Check sheet for the modelled part. Datum: model origin and axes. Units: mm. Give positions to 0.01 mm unless a question says otherwise; leave off trailing zeros. Write each loop counter-clockwise with the first axis right and the second up, starting at its lowest first coordinate (ties: lowest second). Pieces come first, ordered by that corner, then holes. Notation, with made-up numbers: M -27,87 L -18,87 A3 ccw -18,92 Z; hole C 73.5,-17 d3. An arc over 180 degrees is marked long. Write item = value, one per line. Start each with the question number.
1) Gauge pin test, flat end, axial feed: pin 1 (4 mm diameter, centred on x = 60.325, z = -53.975, fed in from +Y). Record the tip position at first contact, or that the pin passes through.
2) Scan lines: L1, parallel to Z at x = 60.5, y = -3 (3 decimals); L2, parallel to X at y = -1, z = -8. Record each from-to range of solid material in increasing order.
3) Draft check along Z on faces 1 (the face through (91, -4, -66.675)), 2 (the face through (62.35, -3.22, -52.42)), 3 (the face through (92.29, -3.78, -33.8)), 4 (the face through (91, -4, 0)). Enter one of: pulls with the +Z half, pulls with the -Z half, needs draft (parallel to the pull), parting line crosses it, or undercut.
4) Sectioned sample at B-B, the plane z = -12.7. Record the cut outline in (x, y) (3 decimals), then the cut area to 3 significant figures.
5) Sectioned sample at C-C, the plane z = -59. Record the cut outline in (x, y) (3 decimals), then the cut area to 3 significant figures.
6) Sectioned sample at A-A, the plane y = -2.5. Count the separate pieces of the cut face and the enclosed holes in it, then the cut area to 3 significant figures.
from build123d import *
from build123d.topology import SkipClean

# Parameters (mm, degrees)
SKETCH1_W              = 184.15
SKETCH1_H              = 66.675
BOSS_EXTRUDE1_DEPTH    = 10.541
SKETCH4_W              = 76.2
SKETCH4_H              = 6.35
BOSS_EXTRUDE2_DEPTH    = 66.675
SKETCH5_W              = 53.975
SKETCH5_H              = 66.675
CUT_EXTRUDE1_DEPTH     = 9.525
SKETCH17_W             = 53.975
SKETCH17_H             = 6.35
BOSS_EXTRUDE3_DEPTH    = 66.675
F_10_CLEARANCE_HOLE1_D = 5.1054
SKETCH12_R             = 31.019294643
CUT_EXTRUDE3_DEPTH     = 197.132329834
SKETCH18_W             = 53.975
SKETCH18_H             = 6.35
BOSS_EXTRUDE4_DEPTH    = 66.675
SKETCH20_W             = 53.975
SKETCH20_H             = 1.016
CUT_EXTRUDE8_DEPTH     = 197.132329834
SKETCH21_R             = 2.5527
CUT_EXTRUDE9_DEPTH     = 197.132329834
SKETCH22_W             = 184.15
SKETCH22_H             = 10.541
CUT_EXTRUDE10_DEPTH    = 197.132329834


with BuildPart() as part:
    # Sketch1 → Boss-Extrude1 (new body)
    with BuildSketch(Plane(origin=(0, 0, 0), x_dir=(1, 0, 0), z_dir=(0, 1, 0))):
        with Locations((92.075, 33.3375)):
            Rectangle(SKETCH1_W, SKETCH1_H)
    extrude(amount=BOSS_EXTRUDE1_DEPTH)

    # Sketch4 → Boss-Extrude2 (add)
    with BuildSketch(Plane.XY):
        with Locations((92.075, -3.175)):
            Rectangle(SKETCH4_W, SKETCH4_H)
    extrude(amount=-BOSS_EXTRUDE2_DEPTH)

    # Sketch5 → Cut-Extrude1 (cut)
    with BuildSketch(Plane(origin=(0, 10.541, 0), x_dir=(1, 0, 0), z_dir=(0, 1, 0))):
        with Locations((92.075, 33.3375)):
            Rectangle(SKETCH5_W, SKETCH5_H)
    extrude(amount=-CUT_EXTRUDE1_DEPTH, mode=Mode.SUBTRACT)

    # Sketch17 → Boss-Extrude3 (add)
    with BuildSketch(Plane.XY):
        with Locations((157.1625, -3.175)):
            Rectangle(SKETCH17_W, SKETCH17_H)
    extrude(amount=-BOSS_EXTRUDE3_DEPTH)

    # #10 Clearance Hole1 (through all)
    with Locations(Plane(origin=(0, 10.541, 0), x_dir=(1, 0, 0), z_dir=(0, 1, 0))):
        with Locations((9.525, 53.975), (9.525, 12.7), (60.325, 12.7), (60.325, 53.975), (123.825, 53.975), (123.849810746, 12.7), (174.625, 12.7), (174.625, 53.975)):
            Hole(F_10_CLEARANCE_HOLE1_D / 2)

    # Sketch12 → Cut-Extrude3 (cut, through all)
    with BuildSketch(Plane(origin=(0, 0, -66.675), x_dir=(-1, 0, 0), z_dir=(0, 0, -1))):
        with Locations((-92.075, 27.239371317)):
            Circle(SKETCH12_R)
    extrude(amount=-CUT_EXTRUDE3_DEPTH, mode=Mode.SUBTRACT)

    # Sketch18 → Boss-Extrude4 (add)
    with BuildSketch(Plane.XY):
        with Locations((26.9875, -3.175)):
            Rectangle(SKETCH18_W, SKETCH18_H)
    extrude(amount=-BOSS_EXTRUDE4_DEPTH)

    # Sketch20 → Cut-Extrude8 (cut, through all)
    with BuildSketch(Plane.XY):
        with Locations((92.075, 0.508)):
            Rectangle(SKETCH20_W, SKETCH20_H)
    extrude(amount=-CUT_EXTRUDE8_DEPTH, mode=Mode.SUBTRACT)

    # Sketch21 → Cut-Extrude9 (cut, through all)
    with SkipClean():  # the faces are left unmerged after this step: merging them gives an invalid solid
        with BuildSketch(Plane(origin=(0, 0, 0), x_dir=(1, 0, 0), z_dir=(0, 1, 0))):
            with Locations(Location((9.525, 12.7, 0), (0, 0, 270))):
                Circle(SKETCH21_R)
            with Locations(Location((9.525, 53.975, 0), (0, 0, 270))):
                Circle(SKETCH21_R)
        extrude(amount=-CUT_EXTRUDE9_DEPTH, mode=Mode.SUBTRACT)

    # Sketch22 → Cut-Extrude10 (cut, through all)
    with BuildSketch(Plane.XY):
        with Locations((92.075, 5.2705)):
            Rectangle(SKETCH22_W, SKETCH22_H)
    extrude(amount=-CUT_EXTRUDE10_DEPTH, mode=Mode.SUBTRACT)


solid = part.part
Data:
q1.pin_1 = through
q2.L1 = -66.675 to -56.522, -51.428 to -15.247, -10.153 to 0
q2.L2 = 0 to 79.24, 104.91 to 184.15
q3.face_1 = pulls with the -Z half
q3.face_2 = undercut
q3.face_3 = needs draft
q3.face_4 = pulls with the +Z half
q4.outline = M 0,-6.35 L 6.972,-6.35 L 6.972,0 L 0,0 Z; M 12.078,-6.35 L 57.772,-6.35 L 57.772,0 L 12.078,0 Z; M 62.878,-6.35 L 121.297,-6.35 L 121.297,0 L 106.915,0 A31.019 cw 77.235,0 L 62.878,0 Z; M 126.403,-6.35 L 172.072,-6.35 L 172.072,0 L 126.403,0 Z; M 177.178,-6.35 L 184.15,-6.35 L 184.15,0 L 177.178,0 Z
q4.area = 964 mm2
q5.outline = M 0,-6.35 L 184.15,-6.35 L 184.15,0 L 106.915,0 A31.019 cw 77.235,0 L 0,0 Z
q5.area = 1,090 mm2
q6.separate_pieces = 2
q6.enclosed_holes = 8
q6.area = 10,900 mm2
